```python
from build123d import *

# Parameters (mm, degrees)
SKETCH1_W           = 88.9
SKETCH1_H           = 88.9
BOSS_EXTRUDE1_DEPTH = 6.35
SKETCH3_W           = 12.7
SKETCH3_H           = 12.7
BOSS_EXTRUDE3_DEPTH = 6.35
SKETCH4_R           = 3.175
CUT_EXTRUDE1_DEPTH  = 7.35
SKETCH6_W           = 12.7
SKETCH6_H           = 12.7
SKETCH6_W_2         = 9.525
SKETCH6_H_2         = 9.525
CUT_EXTRUDE2_DEPTH  = 6.35


with BuildPart() as part:
    # Sketch1 → Boss-Extrude1 (new body)
    with BuildSketch(Plane(origin=(0, 0, 0), x_dir=(1, 0, 0), z_dir=(0, 1, 0))):
        with Locations((38.1, 38.1)):
            Rectangle(SKETCH1_W, SKETCH1_H)
    extrude(amount=BOSS_EXTRUDE1_DEPTH)

    # Sketch3 → Boss-Extrude3 (add)
    with BuildSketch(Plane(origin=(0, 6.35, 0), x_dir=(1, 0, 0), z_dir=(0, 1, 0))):
        with Locations((88.9, 38.1)):
            Rectangle(SKETCH3_W, SKETCH3_H)
        with Locations((-12.7, 38.1)):
            Rectangle(SKETCH3_W, SKETCH3_H)
    extrude(amount=-BOSS_EXTRUDE3_DEPTH)

    # Sketch4 → Cut-Extrude1 (cut, through all)
    with BuildSketch(Plane(origin=(0, 6.35, 0), x_dir=(1, 0, 0), z_dir=(0, 1, 0))):
        with Locations((88.9, 38.1)):
            Circle(SKETCH4_R)
        with Locations((-12.7, 38.1)):
            Circle(SKETCH4_R)
    extrude(amount=-CUT_EXTRUDE1_DEPTH, mode=Mode.SUBTRACT)

    # Sketch6 → Cut-Extrude2 (cut)
    with BuildSketch(Plane(origin=(0, 6.35, 0), x_dir=(1, 0, 0), z_dir=(0, 1, 0))):
        with Locations((20.32, 38.1)):
            Rectangle(SKETCH6_W, SKETCH6_H)
        with Locations((56.8325, 49.2125)):
            Rectangle(SKETCH6_W_2, SKETCH6_H_2)
    extrude(amount=-CUT_EXTRUDE2_DEPTH, mode=Mode.SUBTRACT)


solid = part.part
```
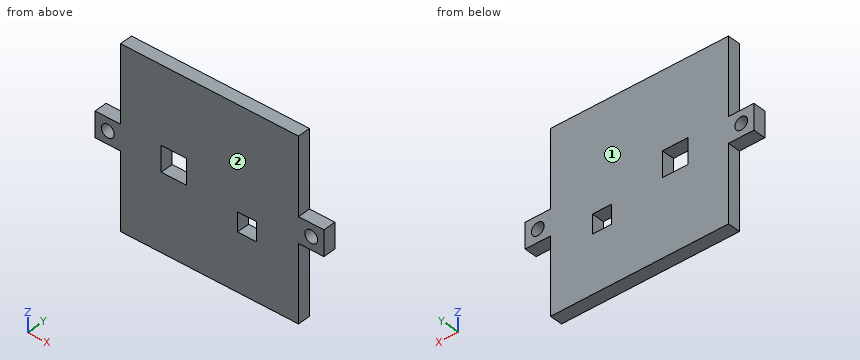
For this review, take the finished solid that the model builds, in its own axes (mm). Face numbers are marked on the shaded views. Round coordinates to 2 decimals unless told otherwise and drop trailing zeros. Loops run counter-clockwise (first coordinate to the right, second up) from the corner with the lowest first, then second, coordinate; pieces in that order, holes last.
(1) Clearance check with flat-ended pins moving along their axes: P1, Ø1.9, axis at y = 2, z = -21.5, coming from the +X side; P2, Ø3, axis at x = 86, y = 4, coming from the -Z side; P3, Ø3, axis at x = -10, y = 2.5, coming from the +Z side. State where each tip first meets the part, or that it passes through.
Returned:
P1: stops at x = 82.55
P2: stops at z = -44.45
P3: stops at z = -31.75
(2) We need section D-D (y = 4). Give the boundary of the cut face in (x, z) (3 decimals).
Returned:
outline: (-19.05, -44.45) - (-6.35, -44.45) - (-6.35, -82.55) - (82.55, -82.55) - (82.55, -44.45) - (95.25, -44.45) - (95.25, -31.75) - (82.55, -31.75) - (82.55, 6.35) - (-6.35, 6.35) - (-6.35, -31.75) - (-19.05, -31.75) - close; hole circle Ø6.35 at (-12.7, -38.1); hole (13.97, -44.45) - (26.67, -44.45) - (26.67, -31.75) - (13.97, -31.75) - close; hole (52.07, -53.975) - (61.595, -53.975) - (61.595, -44.45) - (52.07, -44.45) - close; hole circle Ø6.35 at (88.9, -38.1)
(3) We need section B-B (x = 88.9). Give the boundary of the cut face in (y, z) (3 decimals), plus the area to 3 significant figures.
Returned:
outline: (0, -44.45) - (6.35, -44.45) - (6.35, -41.275) - (0, -41.275) - close; (0, -34.925) - (6.35, -34.925) - (6.35, -31.75) - (0, -31.75) - close
area: 40.3 mm2
(4) Wall thickness on line 1 along X through (y, z) = (3.5, -38.1) (3 decimals); line 2 along X through (y, z) = (2.5, -53.5) (3 decimals); line 3 along Z through (x, y) = (-12.7, 2) (3 decimals): over which ranges is each line inside the solid? List them lowest first.
Returned:
line 1: x = -19.05 to -15.875, -9.525 to 13.97, 26.67 to 85.725, 92.075 to 95.25
line 2: x = -6.35 to 52.07, 61.595 to 82.55
line 3: z = -44.45 to -41.275, -34.925 to -31.75
(5) Mouldability with a two-part tool opening along Y and no side actions: class the marked faces 1 and 2 as released by +Y, released by -Y, zero draft, split by the parting line, or undercut.
Returned:
face 1: released by +Y
face 2: released by -Y
(6) We need section C-C (z = -38.1). Give the boundary of the cut face in (x, y) (3 decimals), plus the area to 3 significant figures.
Returned:
outline: (-19.05, 0) - (-15.875, 0) - (-15.875, 6.35) - (-19.05, 6.35) - close; (-9.525, 0) - (13.97, 0) - (13.97, 6.35) - (-9.525, 6.35) - close; (26.67, 0) - (85.725, 0) - (85.725, 6.35) - (26.67, 6.35) - close; (92.075, 0) - (95.25, 0) - (95.25, 6.35) - (92.075, 6.35) - close
area: 565 mm2
(7) We need section A-A (z = -52). Give the boundary of the cut face in (x, y) (3 decimals), plus the area to 3 significant figures.
Returned:
outline: (-6.35, 0) - (52.07, 0) - (52.07, 6.35) - (-6.35, 6.35) - close; (61.595, 0) - (82.55, 0) - (82.55, 6.35) - (61.595, 6.35) - close
area: 504 mm2
